from build123d import *

# Parameters (mm, degrees)
SKETCH1_W                            = 150
SKETCH1_H                            = 210
SKETCH1_R                            = 2.98
SKETCH1_R_2                          = 3.75
BOSS_EXTRUDE1_DEPTH                  = 6.35
SKETCH2_R                            = 7.9577
CUT_EXTRUDE1_DEPTH                   = 3.175
F_15_64_0_23438_DIAMETER_HOLE1_D     = 6.1849
F_15_64_0_23438_DIAMETER_HOLE1_DEPTH = 7.35
F_15_64_0_23438_DIAMETER_HOLE1_TIP   = 1.858131421
CHAMFER1_SIZE                        = 0.5
SKETCH6_R                            = 7.9577
CUT_EXTRUDE2_DEPTH                   = 3.175
CHAMFER2_SIZE                        = 0.5


with BuildPart() as part:
    # Sketch1 → Boss-Extrude1 (new body)
    with BuildSketch(Plane.XY):
        with Locations((75, 105)):
            Rectangle(SKETCH1_W, SKETCH1_H)
        with Locations((25, 202.5)):
            Circle(SKETCH1_R, mode=Mode.SUBTRACT)
        with Locations((125, 202.5)):
            Circle(SKETCH1_R, mode=Mode.SUBTRACT)
        with Locations((42.5, 202.5)):
            Circle(SKETCH1_R_2, mode=Mode.SUBTRACT)
        with Locations((107.5, 202.5)):
            Circle(SKETCH1_R_2, mode=Mode.SUBTRACT)
        with Locations((107.5, 39)):
            Circle(SKETCH1_R, mode=Mode.SUBTRACT)
        with Locations((42.5, 39)):
            Circle(SKETCH1_R, mode=Mode.SUBTRACT)
        with Locations((42.5, 19)):
            Circle(SKETCH1_R_2, mode=Mode.SUBTRACT)
        with Locations((107.5, 19)):
            Circle(SKETCH1_R_2, mode=Mode.SUBTRACT)
    extrude(amount=BOSS_EXTRUDE1_DEPTH)

    # Sketch2 → Cut-Extrude1 (cut)
    with BuildSketch(Plane.XY.offset(6.35)):
        with Locations((75, 133.75)):
            Circle(SKETCH2_R)
    extrude(amount=-CUT_EXTRUDE1_DEPTH, mode=Mode.SUBTRACT)

    # 15/64 (0.23438) Diameter Hole1
    with Locations(Plane(origin=(25, 183.75, 6.35), x_dir=(1, 0, 0), z_dir=(0, 0, 1))):
        with Locations((0, 0), (100, 0), (100, -100), (0, -100)):
            Hole(F_15_64_0_23438_DIAMETER_HOLE1_D / 2, depth=F_15_64_0_23438_DIAMETER_HOLE1_DEPTH)
            with Locations((0, 0, -(F_15_64_0_23438_DIAMETER_HOLE1_DEPTH + F_15_64_0_23438_DIAMETER_HOLE1_TIP / 2))):  # 118° drill point
                Cone(0, F_15_64_0_23438_DIAMETER_HOLE1_D / 2, F_15_64_0_23438_DIAMETER_HOLE1_TIP, mode=Mode.SUBTRACT)

    # Chamfer1
    chamfer1_edges = [part.edges().sort_by_distance(p)[0] for p in [
        (0, 105, 6.35),
        (104.52, 39, 0),
        (104.52, 39, 6.35),
        (75, 0, 6.35),
        (22.02, 202.5, 0),
        (22.02, 202.5, 6.35),
        (122.02, 202.5, 0),
        (122.02, 202.5, 6.35),
        (38.75, 202.5, 0),
        (38.75, 202.5, 6.35),
        (103.75, 202.5, 0),
        (103.75, 202.5, 6.35),
        (39.52, 39, 0),
        (39.52, 39, 6.35),
        (38.75, 19, 0),
        (38.75, 19, 6.35),
        (103.75, 19, 0),
        (103.75, 19, 6.35),
        (150, 105, 6.35),
        (75, 0, 0),
        (67.0423, 133.75, 6.35),
        (0, 105, 0),
        (75, 210, 0),
        (150, 105, 0),
        (75, 210, 6.35),
        (150, 0, 3.175),
        (0, 0, 3.175),
        (0, 210, 3.175),
        (150, 210, 3.175),
    ]]
    chamfer(chamfer1_edges, length=CHAMFER1_SIZE)

    # Sketch6 → Cut-Extrude2 (cut)
    with BuildSketch(Plane.XY.offset(6.35)):
        with Locations((125, 133.75)):
            Circle(SKETCH6_R)
        with Locations((25, 133.75)):
            Circle(SKETCH6_R)
    extrude(amount=-CUT_EXTRUDE2_DEPTH, mode=Mode.SUBTRACT)

    # Chamfer2
    chamfer2_edges = [part.edges().sort_by_distance(p)[0] for p in [
        (117.0423, 133.75, 6.35),
        (17.0423, 133.75, 6.35),
    ]]
    chamfer(chamfer2_edges, length=CHAMFER2_SIZE)


solid = part.part
Geometry check sheet. Reference: the model listing, model coordinates, mm. A direction names the side the tool comes from. Give positions to 0.01 mm unless a question says otherwise; leave off trailing zeros. Order: outer loops, then holes, each group sorted by start corner. A loop starts at its lowest first (then second) coordinate and runs counter-clockwise, first axis right, second up. Notation, with made-up numbers: M 21.25,-25.75 L 59.25,-25.75 A15 ccw 59.25,-5.75 Z; hole C -35,41.5 d9. An arc over 180 degrees is marked long. Use a Markdown table: item, result.
Item 1: Tool access check on faces 1 (the flat face through (75, 134, 3.175)), 2 (the cylindrical face through (123.57, 181.01, 3.13)). Record the directions out of +Z, -Z, +X, -X, +Y, -Y that give a thin tool (end or side, any length) a straight path to the whole face; none if there is none.
Answers follow:
| item | result |
|---|---|
| face 1 | +Z |
| face 2 | +Z, -Z |
Item 2: Draft check along Y on faces 3 (the flat face through (74, 106, 6.35)), 4 (the flat face through (74, 0, 3)), 5 (the cylindrical face through (107.112, 41.955, 3.138)). Enter one of: +Y half, -Y half, draft (parallel to the pull), parting line (faces both ways), or undercut.
Answers follow:
| item | result |
|---|---|
| face 3 | draft |
| face 4 | -Y half |
| face 5 | undercut |
Item 3: Section check C-C (x = 75). Record the cut outline in (y, z) (3 decimals), and give its area (3 significant figures).
Answers follow:
| item | result |
|---|---|
| outline | M 0,0.5 L 0.5,0 L 209.5,0 L 210,0.5 L 210,5.85 L 209.5,6.35 L 142.208,6.35 L 141.708,5.85 L 141.708,3.175 L 125.792,3.175 L 125.792,5.85 L 125.292,6.35 L 0.5,6.35 L 0,5.85 Z |
| area | 1,280 mm2 |
Item 4: Section check A-A (x = 107.5). State how many separate pieces and enclosed holes the cut face has, and give its area (3 significant figures).
Answers follow:
| item | result |
|---|---|
| separate pieces | 4 |
| enclosed holes | 0 |
| area | 1,200 mm2 |
Item 5: Depth check by flat-ended pin: P1, Ø8, axis at x = 125, y = 83.75, coming from the +Z side; P2, Ø5, axis at x = 123.5, y = 136, coming from the +Z side (3 decimals); P3, Ø5.5, axis at x = 42.5, y = 39, coming from the +Z side. Enter the tip coordinate at first touch or a pass-through.
Answers follow:
| item | result |
|---|---|
| P1 | stops at z = 6.35 |
| P2 | stops at z = 3.175 |
| P3 | passes through |
Item 6: Material ranges on line 1 along X through (y, z) = (183.75, 5); line 2 along X through (y, z) = (184.5, 1.25); line 3 along Y through (x, z) = (25, 2.75), recorded low to high.
Answers follow:
| item | result |
|---|---|
| line 1 | x = 0 to 21.91, 28.09 to 121.91, 128.09 to 150 |
| line 2 | x = 0 to 22, 28 to 122, 128 to 150 |
| line 3 | y = 0 to 80.66, 86.84 to 180.66, 186.84 to 199.52, 205.48 to 210 |
